from build123d import *

# Parameters (mm, degrees)
SKETCH_1_W               = 555
SKETCH_1_H               = 50
EXTRUDE_1_DEPTH          = 20
SKETCH_2_R               = 15
CUT_EXTRUDE_1_DEPTH      = 280.340741747
CUT_EXTRUDE_2_REACH      = 557.923
CUT_EXTRUDE_2_END_RADIUS = 15
SKETCH_3_R               = 6
FILLET_1_R               = 10
CHAMFER_1_SIZE           = 0.5


with BuildPart() as part:
    # 草图1 → 凸台-拉伸1 (new body)
    with BuildSketch(Plane(origin=(0, 0, 0), x_dir=(1, 0, 0), z_dir=(0, 1, 0))):
        Rectangle(SKETCH_1_W, SKETCH_1_H)
    extrude(amount=EXTRUDE_1_DEPTH)

    # 草图2 → 切除-拉伸1 (cut, through all)
    with BuildSketch(Plane(origin=(0, 20, 0), x_dir=(1, 0, 0), z_dir=(0, 1, 0))):
        with Locations(Location((-242.5, 0, 0), (0, 0, 270))):
            Circle(SKETCH_2_R)
        with Locations(Location((-172.5, 0, 0), (0, 0, 270))):
            Circle(SKETCH_2_R)
        with Locations(Location((-102.5, 0, 0), (0, 0, 270))):
            Circle(SKETCH_2_R)
        with BuildLine():
            Line((81.5, 15), (241.5, 15))
            ThreePointArc((241.5, 15), (256.5, 0), (241.5, -15))
            Line((241.5, -15), (81.5, -15))
            ThreePointArc((81.5, -15), (66.5, 0), (81.5, 15))
        make_face()
    extrude(amount=-CUT_EXTRUDE_1_DEPTH, mode=Mode.SUBTRACT)

    # 切除-拉伸2: up to this cylinder (the profile starts outside it)
    cut_extrude_2_end = Plane(origin=(241.5, 10, 0), z_dir=(0, 1, 0)) * Cylinder(CUT_EXTRUDE_2_END_RADIUS, 1146.846, mode=Mode.PRIVATE)
    # 草图3 → 切除-拉伸2 (cut, up to the surface)
    with BuildSketch(Plane(origin=(277.5, 0, 0), x_dir=(0, 0, -1), z_dir=(1, 0, 0)), mode=Mode.PRIVATE) as cut_extrude_2_sk1:
        with Locations((0, 10)):
            Circle(SKETCH_3_R)
    cut_extrude_2_tool1 = extrude(cut_extrude_2_sk1.sketch, amount=-CUT_EXTRUDE_2_REACH, mode=Mode.PRIVATE) - cut_extrude_2_end
    add(cut_extrude_2_tool1.solids().sort_by_distance((277.5, 10, 0))[0], mode=Mode.SUBTRACT)

    # 圆角1
    fillet_1_edges = [part.edges().sort_by_distance(p)[0] for p in [
        (-277.5, 10, -25),
        (277.5, 10, -25),
        (277.5, 10, 25),
        (-277.5, 10, 25),
    ]]
    fillet(fillet_1_edges, radius=FILLET_1_R)

    # 倒角1
    chamfer_1_edges = [part.edges().sort_by_distance(p)[0] for p in [
        (-242.5, 0, -15),
        (-242.5, 20, -15),
        (-172.5, 0, -15),
        (-172.5, 20, -15),
        (-102.5, 0, -15),
        (-102.5, 20, -15),
        (66.5, 0, 0),
        (161.5, 0, -15),
        (256.5, 0, 0),
        (161.5, 0, 15),
        (66.5, 20, 0),
        (161.5, 20, 15),
        (256.5, 20, 0),
        (161.5, 20, -15),
    ]]
    chamfer(chamfer_1_edges, length=CHAMFER_1_SIZE)


solid = part.part
Design review of the part built by this model. Coordinates are the model's own, in mm. A direction names the side the tool comes from. Round coordinates to 2 decimals unless told otherwise and drop trailing zeros. Write each loop counter-clockwise with the first axis right and the second up, starting at its lowest first coordinate (ties: lowest second). Pieces come first, ordered by that corner, then holes. Notation, with made-up numbers: (73.5, -24) -> (104.5, -24) arc R24 ccw to (104.5, 12) -> close; hole circle Ø5 at (15, 86.25). An arc over 180 degrees is marked (long way). One line per item, written item: value. Start each with the question number.
Q1. To check wall thickness, follow probe 1 along X at (y, z) = (2, -0.5); probe 2 along X at (y, z) = (15.5, 0); probe 3 along Y at (x, z) = (261.5, 0). State the ranges of each line that lie inside material, in increasing order.
Q2. Tool access review of faces 1 (the face through (255.705, 14.355, 4.819)), 2 (the face through (266.529, 4.143, 1.301)), 3 (the face through (66.368, 0.365, -0.333)): name each direction out of +Z, -Z, +X, -X, +Y, -Y from which nothing blocks a thin tool from reaching the whole face with its end or side.
Q3. Add section C-C (z = 0). State how many separate pieces and enclosed holes the cut face has, then the cut area to 3 significant figures.
Q4. Add section A-A (x = -172.5). Give the boundary of the cut face in (y, z).
Q5. Add section B-B (y = 10). Give the boundary of the cut face in (x, z), then the cut area to 3 significant figures.
Q6. The part is to be moulded in two halves that separate along Z. For faces 4 (the face through (256.632, 0.365, 0.333)), 5 (the face through (-274.65, 10.14, 21.99)), 6 (the face through (274.49, 10.14, -22.15)), say which applies: pulls with the +Z half, pulls with the -Z half, needs draft (parallel to the pull), parting line crosses it, or undercut.
Response:
1. probe 1: x = -277.5 to -257.49, -227.51 to -187.49, -157.51 to -117.49, -87.51 to 66.51, 256.49 to 277.5
1. probe 2: x = -277.5 to -257.5, -227.5 to -187.5, -157.5 to -117.5, -87.5 to 66.5
1. probe 3: y = 0 to 4, 16 to 20
2. face 1: +Y, -Y
2. face 2: +X
2. face 3: -Y
3. separate pieces: 6
3. enclosed holes: 0
3. area: 5,250 mm^2
4. outline: (0, -25) -> (20, -25) -> (20, -15.5) -> (19.5, -15) -> (0.5, -15) -> (0, -15.5) -> close; (0, 15.5) -> (0.5, 15) -> (19.5, 15) -> (20, 15.5) -> (20, 25) -> (0, 25) -> close
5. outline: (-277.5, -15) arc R10 ccw to (-267.5, -25) -> (267.5, -25) arc R10 ccw to (277.5, -15) -> (277.5, -6) -> (255.25, -6) arc R15 cw to (241.5, -15) -> (81.5, -15) arc R15 cw to (81.5, 15) -> (241.5, 15) arc R15 cw to (255.25, 6) -> (277.5, 6) -> (277.5, 15) arc R10 ccw to (267.5, 25) -> (-267.5, 25) arc R10 ccw to (-277.5, 15) -> close; hole circle Ø30 at (-242.5, 0); hole circle Ø30 at (-172.5, 0); hole circle Ø30 at (-102.5, 0)
5. area: 19,800 mm^2
6. face 4: undercut
6. face 5: pulls with the +Z half
6. face 6: pulls with the -Z half
